from build123d import *
from build123d.topology import SkipClean

# Parameters (mm, degrees)
SKETCH_1_R          = 210
SKETCH_1_R_2        = 203
EXTRUDE_2_DEPTH     = 174
EXTRUDE_START       = -174
EXTRUDE_4_DEPTH     = 174
CUT_EXTRUDE_1_DEPTH = 654
EXTRUDE_5_DEPTH     = 174
EXTRUDE_6_DEPTH     = 174
EXTRUDE_7_DEPTH     = 174
EXTRUDE_8_DEPTH     = 174
CUT_EXTRUDE_START   = -654
CUT_EXTRUDE_2_DEPTH = 654
SKETCH_10_W         = 20.487801248
SKETCH_10_H         = 174
CUT_EXTRUDE_3_DEPTH = 327
SKETCH_11_W         = 235.63772895
SKETCH_11_H         = 249.192111589
CUT_EXTRUDE_4_DEPTH = 238
EXTRUDE_10_DEPTH    = 180
SKETCH_17_W         = 286.098661696
SKETCH_17_H         = 191.878669743
CUT_EXTRUDE_5_DEPTH = 322
EXTRUDE_11_DEPTH    = 180
SKETCH_20_R         = 4
CUT_EXTRUDE_7_DEPTH = 555.5


with BuildPart() as part:
    # 草图1 → 凸台-拉伸2 (new body)
    with BuildSketch(Plane.XY):
        Circle(SKETCH_1_R)
        Circle(SKETCH_1_R_2, mode=Mode.SUBTRACT)
    extrude(amount=EXTRUDE_2_DEPTH)

    # 草图2 → 凸台-拉伸4 (add)
    with BuildSketch(Plane.XY.offset(174).offset(EXTRUDE_START)):
        with BuildLine():
            Line((-170.735431044, -102), (-173.735431044, -102))
            Line((-173.735431044, -102), (-175.513532242, -102))
            ThreePointArc((-175.513532242, -102), (-174.63092392, -103.50381834), (-173.735431044, -105))
            Line((-173.735431044, -105), (-170.735431044, -105))
            Line((-170.735431044, -105), (-170.735431044, -102))
        make_face()
        with BuildLine():
            ThreePointArc((173.735431044, -105), (174.63092392, -103.50381834), (175.513532242, -102))
            Line((175.513532242, -102), (173.735431044, -102))
            Line((173.735431044, -102), (170.735431044, -102))
            Line((170.735431044, -102), (170.735431044, -105))
            Line((170.735431044, -105), (173.735431044, -105))
        make_face()
    extrude(amount=EXTRUDE_4_DEPTH)

    # 草图3 → 切除-拉伸1 (cut)
    with BuildSketch(Plane.XY.offset(174)):
        Polygon((-170.735431044, -102), (238.333646515, -102), (254.334169784, 272.292523591), (-334.569415043, 221.85110305), (-306.830562533, -102), align=None)
    extrude(amount=-CUT_EXTRUDE_1_DEPTH, mode=Mode.SUBTRACT)

    # 草图5 → 凸台-拉伸5 (add)
    with BuildSketch(Plane.XY.offset(174).offset(EXTRUDE_START)):
        with BuildLine():
            Line((-120, -209.75), (-10.243900624, -209.75))
            ThreePointArc((-10.243900624, -209.75), (-67.755470707, -198.769203322), (-120, -172.336879396))
            Line((-120, -172.336879396), (-120, -209.75))
        make_face()
        with BuildLine():
            ThreePointArc((120, -172.336879396), (67.755470707, -198.769203322), (10.243900624, -209.75))
            Line((10.243900624, -209.75), (120, -209.75))
            Line((120, -209.75), (120, -172.336879396))
        make_face()
    extrude(amount=EXTRUDE_5_DEPTH)

    # 草图6 → 凸台-拉伸6 (add)
    with BuildSketch(Plane.XY.offset(174).offset(EXTRUDE_START)):
        with BuildLine():
            Line((-175.513532242, -102), (-166.195667814, -102))
            ThreePointArc((-166.195667814, -102), (0, -195), (166.195667814, -102))
            Line((166.195667814, -102), (175.513532242, -102))
            ThreePointArc((175.513532242, -102), (0, -203), (-175.513532242, -102))
        make_face()
    extrude(amount=EXTRUDE_6_DEPTH)

    # 草图7 → 凸台-拉伸7 (add)
    with BuildSketch(Plane.XY.offset(174).offset(EXTRUDE_START)):
        with BuildLine():
            Line((-166.933126535, -92), (-166.933126535, -95))
            Line((-166.933126535, -95), (-170.293863659, -95))
            ThreePointArc((-170.293863659, -95), (0, -195), (170.293863659, -95))
            Line((170.293863659, -95), (166.933126535, -95))
            Line((166.933126535, -95), (166.933126535, -92))
            Line((166.933126535, -92), (171.933126535, -92))
            Line((171.933126535, -92), (188.496850106, -92))
            ThreePointArc((188.496850106, -92), (0, -209.75), (-188.496850106, -92))
            Line((-188.496850106, -92), (-171.933126535, -92))
            Line((-171.933126535, -92), (-166.933126535, -92))
        make_face()
    extrude(amount=EXTRUDE_7_DEPTH)

    # 草图8 → 凸台-拉伸8 (add)
    with BuildSketch(Plane(origin=(0, 0, 0), x_dir=(-1, 0, 0), z_dir=(0, 0, -1))):
        with BuildLine():
            Line((166.933126535, -92), (163.933126535, -92))
            Line((163.933126535, -92), (163.933126535, -99))
            Line((163.933126535, -99), (168, -99))
            ThreePointArc((168, -99), (169.158755456, -97.006780447), (170.293863659, -95))
            Line((170.293863659, -95), (166.933126535, -95))
            Line((166.933126535, -95), (166.933126535, -92))
        make_face()
        with BuildLine():
            Line((-166.933126535, -95), (-170.293863659, -95))
            ThreePointArc((-170.293863659, -95), (-169.158755456, -97.006780447), (-168, -99))
            Line((-168, -99), (-163.933126535, -99))
            Line((-163.933126535, -99), (-163.933126535, -92))
            Line((-163.933126535, -92), (-166.933126535, -92))
            Line((-166.933126535, -92), (-166.933126535, -95))
        make_face()
    extrude(amount=-EXTRUDE_8_DEPTH)

    # 草图9 → 切除-拉伸2 (cut)
    with BuildSketch(Plane.XY.offset(174).offset(CUT_EXTRUDE_START)):
        with BuildLine():
            Line((0, -195), (0, -182.225251044))
            Line((0, -182.225251044), (-50, -182.225251044))
            Line((-50, -182.225251044), (-50, -188.48076825))
            ThreePointArc((-50, -188.48076825), (-25.211606368, -193.363323576), (0, -195))
        make_face()
        with BuildLine():
            Line((0, -209.75), (0, -195))
            ThreePointArc((0, -195), (-25.211606368, -193.363323576), (-50, -188.48076825))
            Line((-50, -188.48076825), (-50, -195))
            Line((-50, -195), (-50, -209.75))
            Line((-50, -209.75), (-10.243900624, -209.75))
            Line((-10.243900624, -209.75), (0, -209.75))
        make_face()
        with BuildLine():
            ThreePointArc((50, -188.48076825), (25.211606368, -193.363323576), (0, -195))
            Line((0, -195), (0, -209.75))
            Line((0, -209.75), (10.243900624, -209.75))
            Line((10.243900624, -209.75), (50, -209.75))
            Line((50, -209.75), (50, -195))
            Line((50, -195), (50, -188.48076825))
        make_face()
        with BuildLine():
            Line((50, -182.225251044), (0, -182.225251044))
            Line((0, -182.225251044), (0, -195))
            ThreePointArc((0, -195), (25.211606368, -193.363323576), (50, -188.48076825))
            Line((50, -188.48076825), (50, -182.225251044))
        make_face()
    extrude(amount=CUT_EXTRUDE_2_DEPTH, mode=Mode.SUBTRACT)


with BuildPart() as cut_extrude_2_piece_1:
    # of the separate pieces the step leaves, piece 1, a body of its own (cut_extrude_2_pieces)
    add(part.part.solids().sort_by_distance((-183.564702489, -102, 0))[0])

    # 草图11 → 切除-拉伸4 (cut)
    with BuildSketch(Plane(origin=(0, 0, 0), x_dir=(-1, 0, 0), z_dir=(0, 0, -1))):
        with Locations((136.586471206, -141.23053543)):
            Rectangle(SKETCH_11_W, SKETCH_11_H)
    extrude(amount=-CUT_EXTRUDE_4_DEPTH, mode=Mode.SUBTRACT)


with BuildPart() as cut_extrude_2_piece_2:
    # of the separate pieces the step leaves, piece 2, a body of its own (cut_extrude_2_pieces)
    add(part.part.solids().sort_by_distance((50, -188.48076825, 0))[0])

    # 草图17 → 切除-拉伸5 (cut)
    with BuildSketch(Plane(origin=(0, -92, 0), x_dir=(1, 0, 0), z_dir=(0, 1, 0))):
        with Locations((123.864076708, -90.777636372)):
            Rectangle(SKETCH_17_W, SKETCH_17_H)
    extrude(amount=-CUT_EXTRUDE_5_DEPTH, mode=Mode.SUBTRACT)


with BuildPart() as cut_extrude_2_piece_3:
    # of the separate pieces the step leaves, piece 3, a body of its own (cut_extrude_2_pieces)
    add(part.part.solids().sort_by_distance((10.243900624, -209.75, 0))[0])

    # 草图10 → 切除-拉伸3 (cut, symmetric)
    with BuildSketch(Plane(origin=(0, -209.75, 0), x_dir=(1, 0, 0), z_dir=(0, 1, 0))):
        with Locations((0, -87)):
            Rectangle(SKETCH_10_W, SKETCH_10_H)
    extrude(amount=CUT_EXTRUDE_3_DEPTH, both=True, mode=Mode.SUBTRACT)


with BuildPart() as body_2:
    # 草图14 → 凸台-拉伸10 (new body)
    with BuildSketch(Plane.XY.offset(209.75)):
        with BuildLine():
            Line((0, 210), (0, 205))
            ThreePointArc((0, 205), (174.477792283, 107.622023768), (183.196615689, -92))
            Line((183.196615689, -92), (188.774998345, -92))
            ThreePointArc((188.774998345, -92), (178.073018731, 111.310376875), (0, 210))
        make_face()
    extrude(amount=EXTRUDE_10_DEPTH)

    # 草图18 → 凸台-拉伸11 (add)
    with SkipClean():  # the faces are left unmerged after this step: merging them gives an invalid solid
        with BuildSketch(Plane.XY.offset(389.75)):
            with BuildLine():
                ThreePointArc((0, 210), (-178.073018731, 111.310376875), (-188.774998345, -92))
                Line((-188.774998345, -92), (-183.196615689, -92))
                ThreePointArc((-183.196615689, -92), (-174.477792283, 107.622023768), (0, 205))
                Line((0, 205), (0, 210))
            make_face()
        extrude(amount=-EXTRUDE_11_DEPTH)

    # 草图20 → 切除-拉伸7 (cut, symmetric)
    with SkipClean():  # the faces are left unmerged after this step: merging them gives an invalid solid
        with BuildSketch(Plane(origin=(0, 0, 0), x_dir=(0, 0, -1), z_dir=(1, 0, 0))):
            with Locations((-382.75, 78)):
                Circle(SKETCH_20_R)
        extrude(amount=CUT_EXTRUDE_7_DEPTH, both=True, mode=Mode.SUBTRACT)


solid = body_2.part
CAD build for the part. Positions are in the model's coordinates, mm. Give positions to 0.01 mm unless a question says otherwise; leave off trailing zeros. Write each loop counter-clockwise with the first axis right and the second up, starting at its lowest first coordinate (ties: lowest second). Pieces come first, ordered by that corner, then holes. Notation, with made-up numbers: (5.25, 21) - (54.25, 21) arc R23 ccw to (54.25, 35) - close; hole circle Ø3 at (-20.75, -10). An arc over 180 degrees is marked (long way). Put each result on its own line as item: value.
(1) Saw through at B-B (z = 339.5). List the corners of the cut face in (x, y) (3 decimals), then the cut area to 3 significant figures.
Working result:
outline: (-188.775, -92) - (-183.197, -92) arc R205 cw (long way) to (183.197, -92) - (188.775, -92) arc R210 ccw (long way) to start
area: 4,210 mm^2
(2) Saw through at D-D (x = -9.5). List the corners of the cut face in (y, z) (3 decimals), then the cut area to 3 significant figures.
Working result:
outline: (204.78, 209.75) - (209.785, 209.75) - (209.785, 389.75) - (204.78, 389.75) - close
area: 901 mm^2
(3) Saw through at C-C (y = -40.5). List the corners of the cut face in (x, z).
Working result:
outline: (-206.06, 209.75) - (-200.96, 209.75) - (-200.96, 389.75) - (-206.06, 389.75) - close; (200.96, 209.75) - (206.06, 209.75) - (206.06, 389.75) - (200.96, 389.75) - close
(4) Wall check: L1, parallel to Z at x = -190.75, y = 78; L2, parallel to X at y = 71.5, z = 344.5; L3, parallel to X at y = -40, z = 379.5. Give the ranges that are in metal, low to high.
Working result:
L1: 209.75 to 378.75, 386.75 to 389.75
L2: -197.45 to -192.13, 192.13 to 197.45
L3: -206.16 to -201.06, 201.06 to 206.16
(5) Drop flat-ended pins along their axis: pin 1 Ø5 at (y, z) = (163, 344) entering from -X; pin 2 Ø2 at (y, z) = (52.5, 359) entering from +X; pin 3 Ø5 at (x, z) = (110, 321.5) entering from -Y. Give the stop position or say it passes through.
Working result:
pin 1: x = -135.42
pin 2: x = 203.59
pin 3: y = 171.37
(6) Saw through at A-A (y = 101.5). List the corners of the cut face in (x, z), then the cut area to 3 significant figures.
Working result:
outline: (-183.84, 209.75) - (-178.11, 209.75) - (-178.11, 389.75) - (-183.84, 389.75) - close; (178.11, 209.75) - (183.84, 209.75) - (183.84, 389.75) - (178.11, 389.75) - close
area: 2,060 mm^2
